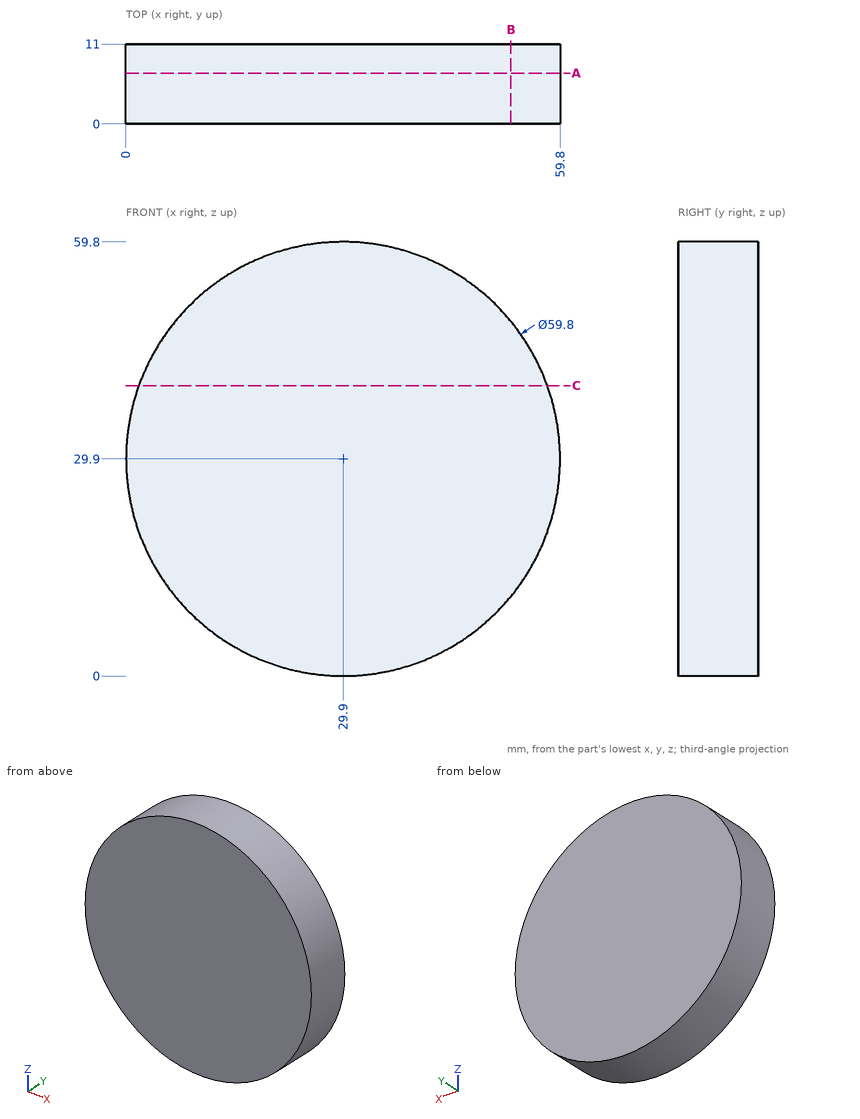
The figure shows three views and two pictorial views of one solid part (mm, origin at its lowest corner). Answer the questions. Coordinates: 2 decimals unless noted, no trailing zeros. Loops run counter-clockwise (first coordinate to the right, second up) from the corner with the lowest first, then second, coordinate; pieces in that order, holes last. Notation, with made-up numbers: (81, 19.25) - (127, 19.25) arc R18 cw to (127, 54.25) - close; hole circle Ø8 at (39, -33.75). An arc over 180 degrees is marked (long way). Answer in a Markdown table with one row per item.
Q1. Find section C-C on z = 40. Write down the section's boundary in (x, y), plus the area to 3 significant figures.
Here are the results:
| item | result |
|---|---|
| outline | (1.76, 0) - (58.04, 0) - (58.04, 11) - (1.76, 11) - close |
| area | 619 mm^2 |
Q2. Find section A-A on y = 7. Write down the section's boundary in (x, z).
Here are the results:
| item | result |
|---|---|
| outline | circle Ø59.8 at (29.9, 29.9) |
Q3. Given P1, Ø1.5, axis at y = 1.5, z = 8, coming from the +X side (3 decimals); P2, Ø2, axis at y = 10, z = 22.5, coming from the -X side; P3, Ø2, axis at y = 7.5, z = 21, coming from the -X side, each flat-ended and moving along its own axis, determine where each tip first touches the part or whether it passes through.
Here are the results:
| item | result |
|---|---|
| P1 | stops at x = 51.035 |
| P2 | stops at x = 0.69 |
| P3 | stops at x = 1.06 |
Q4. Find section B-B on x = 53. Write down the section's boundary in (y, z).
Here are the results:
| item | result |
|---|---|
| outline | (0, 10.92) - (11, 10.92) - (11, 48.88) - (0, 48.88) - close |
Q5. Straight lines are drawn through the part: line 1 along X through (y, z) = (8.75, 25); line 2 along Z through (x, y) = (11, 7.5); line 3 along X through (y, z) = (2.75, 12.5). For each, find the intervals that lie inside material, in ascending order. Write a range as [from, to].
Here are the results:
| item | result |
|---|---|
| line 1 | x = [0.4, 59.4] |
| line 2 | z = [6.73, 53.07] |
| line 3 | x = [5.58, 54.22] |
